For this review, use the dimensioned drawing (mm, ordinates from the lowest corner) and the shaded views. A direction names the side the tool comes from. Coordinates: 2 decimals unless noted, no trailing zeros. Write each loop counter-clockwise with the first axis right and the second up, starting at its lowest first coordinate (ties: lowest second). Pieces come first, ordered by that corner, then holes.
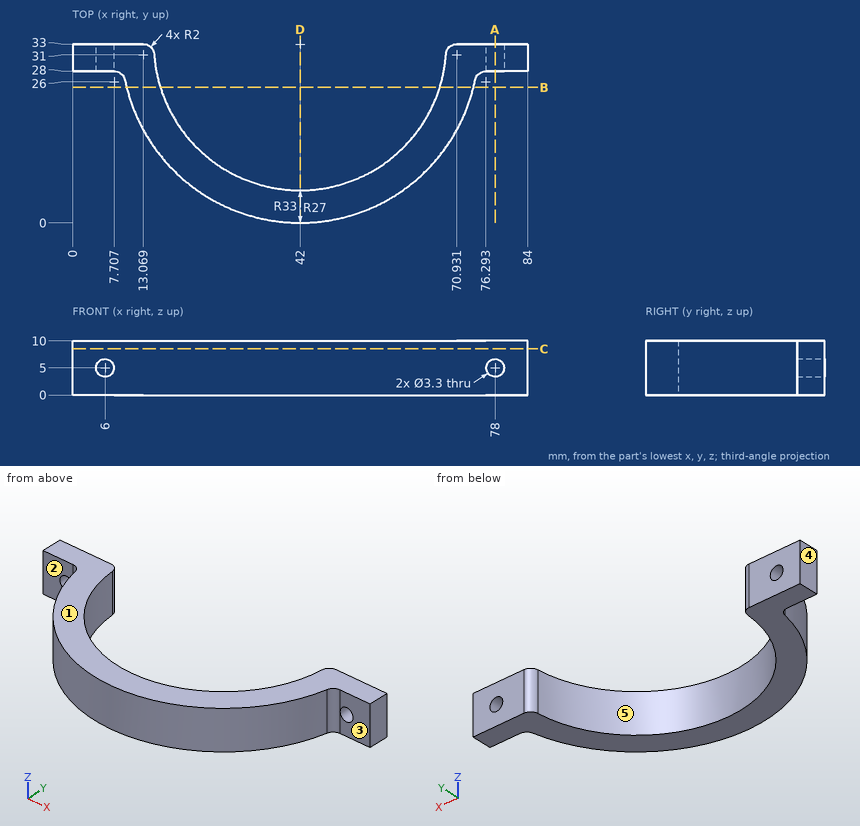
Item 1: Take a section at A-A, the plane x = 78. Write out the cut boundary in (y, z).
Solved:
outline: (28, 0) - (33, 0) - (33, 3.35) - (28, 3.35) - close; (28, 6.65) - (33, 6.65) - (33, 10) - (28, 10) - close
Item 2: Take a section at D-D, the plane x = 42. Write out the cut boundary in (y, z), plus the area to 3 significant figures.
Solved:
outline: (0, 0) - (6, 0) - (6, 10) - (0, 10) - close
area: 60.0 mm2
Item 3: Machinability: for the marked faces 1 and 2, which of the approach directions +Z, -Z, +X, -X, +Y, -Y give a long, thin tool a straight path to every point of the face, cutting with its end or side? Answer none if there is none.
Solved:
face 1: +Z, +X, -X, +Y, -Y
face 2: +Z, -Z, -X, -Y
Item 4: Mouldability with a two-part tool opening along X and no side actions: class the marked faces 3, 4 and 5 as pulls with the +X half, pulls with the -X half, needs draft (parallel to the pull), parting line crosses it, or undercut.
Solved:
face 3: needs draft
face 4: pulls with the -X half
face 5: undercut
Item 5: To check wall thickness, follow line 1 along X through (y, z) = (31.25, 5); line 2 along X through (y, z) = (29, 5); line 3 along Z through (x, y) = (78, 29.55). State the ranges of each line that lie inside material, in increasing order.
Solved:
line 1: x = 0 to 4.35, 7.65 to 15.05, 68.95 to 76.35, 79.65 to 84
line 2: x = 0 to 4.35, 7.65 to 15.3, 68.7 to 76.35, 79.65 to 84
line 3: z = 0 to 3.35, 6.65 to 10
Item 6: Take a section at C-C, the plane z = 8.5. Write out the cut boundary in (x, y).
Solved:
outline: (0, 28) - (7.71, 28) arc R2 cw to (9.67, 26.4) arc R33 ccw to (74.33, 26.4) arc R2 cw to (76.29, 28) - (84, 28) - (84, 33) - (70.93, 33) arc R2 ccw to (68.94, 31.14) arc R27 cw to (15.06, 31.14) arc R2 ccw to (13.07, 33) - (0, 33) - close
Item 7: For pin 1 (3 mm diameter, centred on x = 78, z = 5, fed in from -Y); pin 2 (1 mm diameter, centred on x = 24.5, z = 7, fed in from +Y) (1 decimal); pin 3 (2 mm diameter, centred on x = 33, z = 7, fed in from +Y); pin 4 (5 mm diameter, centred on y = 7.5, z = 2.5, fed in from +X), all flat-tipped, find the tip position at first contact; note any pin that passes through.
Solved:
pin 1: passes through
pin 2: stops at y = 12.9
pin 3: stops at y = 7.92
pin 4: stops at x = 65.66
Item 8: Take a section at B-B, the plane y = 25. Write out the cut boundary in (x, z), plus the area to 3 significant figures.
Solved:
outline: (9.98, 0) - (16.21, 0) - (16.21, 10) - (9.98, 10) - close; (67.79, 0) - (74.02, 0) - (74.02, 10) - (67.79, 10) - close
area: 125 mm2
